Design review of the part built by this model. Coordinates are the model's own, in mm. Face numbers are marked on the shaded views. A direction names the side the tool comes from. Round coordinates to 2 decimals unless told otherwise and drop trailing zeros. Loops run counter-clockwise (first coordinate to the right, second up) from the corner with the lowest first, then second, coordinate; pieces in that order, holes last. Notation, with made-up numbers: (-11, 88.5) - (-1, 88.5) arc R6 cw to (-1, 92.5) - close; hole circle Ø11 at (8, -8.5). An arc over 180 degrees is marked (long way). Answer as CSV lines item,"result". Start each with the question number.
(1) Consider section B-B (x = 0). Give the boundary of the cut face in (y, z).
(2) For the marked faces 1, 2 and 3, list the 3-axis set-ups (+Z, -Z, +X, -X, +Y, -Y) from which the entire face can be reached by the end or side of a thin tool; tool diameter is ignored.
(3) Consider section A-A (y = 0). Give the boundary of the cut face in (x, z), and give its area (3 significant figures).
(4) Wall thickness on L1, parallel to Z at x = -4.5, y = 2.5; L2, parallel to X at y = -2.5, z = 9.5; L3, parallel to Y at x = 1.25, z = 14: over which ranges is each line inside the solid? List them lowest first.
(5) Consider section D-D (y = -3). Give the boundary of the cut face in (x, z), and give its area (3 significant figures).
(6) Consider section C-C (z = -1). Give the boundary of the cut face in (x, y).
(7) For P1, Ø6, axis at x = -5.5, z = -1, coming from the +Y side; P2, Ø2, axis at y = -1, z = 2, coming from the +X side; P3, Ø1.5, axis at y = -2.5, z = 5, coming from the +X side, all flat-tipped, find the tip position at first contact; note any pin that passes through.
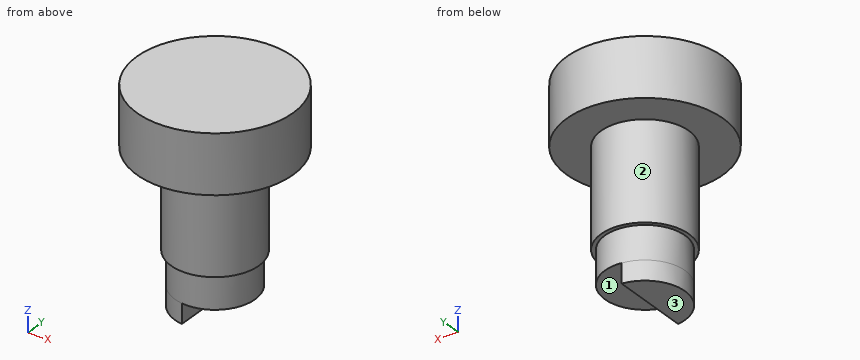
from build123d import *

# Parameters (mm, degrees)
F0_R     = 4.5
F1_DEPTH = 8
F2_R     = 4.5
F3_DEPTH = 2
F4_R     = 8
F5_DEPTH = 6
F6_R     = 4.1
F7_DEPTH = 3.4
F9_DEPTH = 2


# Not quite as in the source:
# - a feature names something its author has since deleted; it is built from what else it names


with BuildPart() as f1:
    # F0 (on Top) → F1 (new body)
    with BuildSketch(Plane.XY):
        Circle(F0_R)
    extrude(amount=F1_DEPTH)

    # F2 (on face) → F3 (join)
    with BuildSketch(Plane.XY.offset(8)):
        Circle(F2_R)
    extrude(amount=F3_DEPTH)

    # F4 (on face) → F5 (join)
    with BuildSketch(Plane.XY.offset(10)):
        Circle(F4_R)
    extrude(amount=F5_DEPTH)

    # F6 (on face) → F7 (join)
    with BuildSketch(Plane(origin=(0, 0, 0), x_dir=(1, 0, 0), z_dir=(0, 0, -1))):
        Circle(F6_R)
    extrude(amount=F7_DEPTH)

    # F8 (on face) → F9 (join)
    with BuildSketch(Plane(origin=(0, 0, -3.4), x_dir=(1, 0, 0), z_dir=(0, 0, -1))):
        with BuildLine():
            Line((-0.499664308, 0), (-0.499664308, 4.0694392217))
            ThreePointArc((-0.499664308, 4.0694392217), (-4.1, 0), (-0.499664308, -4.0694392217))
            Line((-0.499664308, -4.0694392217), (-0.499664308, 0))
        make_face()
    extrude(amount=F9_DEPTH)


solid = f1.part
Determined:
1,outline,"(-8, 10) - (-4.5, 10) - (-4.5, 0) - (-4.1, 0) - (-4.1, -3.4) - (4.1, -3.4) - (4.1, 0) - (4.5, 0) - (4.5, 10) - (8, 10) - (8, 16) - (-8, 16) - close"
2,face 1,"-Z, +X, +Y, -Y"
2,face 2,"-Z"
2,face 3,"-Z, +X, -X, +Y, -Y"
3,outline,"(-8, 10) - (-4.5, 10) - (-4.5, 0) - (-4.1, 0) - (-4.1, -5.4) - (-0.5, -5.4) - (-0.5, -3.4) - (4.1, -3.4) - (4.1, 0) - (4.5, 0) - (4.5, 10) - (8, 10) - (8, 16) - (-8, 16) - close"
3,area,"221 mm^2"
4,L1,"z = 10 to 16"
4,L2,"x = -3.74 to 3.74"
4,L3,"y = -7.9 to 7.9"
5,outline,"(-7.42, 10) - (-3.35, 10) - (-3.35, 0) - (-2.79, 0) - (-2.79, -5.4) - (-0.5, -5.4) - (-0.5, -3.4) - (2.79, -3.4) - (2.79, 0) - (3.35, 0) - (3.35, 10) - (7.42, 10) - (7.42, 16) - (-7.42, 16) - close"
5,area,"180 mm^2"
6,outline,"circle Ø8.2 at (0, 0)"
7,P1,"stops at y = 3.62"
7,P2,"stops at x = 4.5"
7,P3,"stops at x = 4.15"
